Autodesk Inventor part; units mm, degrees
ref_plane "YZ Plane" through (0, 0, 0) normal (1, 0, 0) x (0, 1, 0)
ref_plane "XZ Plane" through (0, 0, 0) normal (0, 1, 0) x (-1, 0, 0)
ref_plane "XY Plane" through (0, 0, 0) normal (0, 0, 1) x (1, 0, 0)
sketch "Sketch1" plane through (0, 0, 0) normal (0, 1, 0) x (-1, 0, 0)
  line L0 (10.1226, -11.6524) -> (10.1226, 93.3476)
  line L1 (-18.8774, 93.3476) -> (-18.8774, -11.6524)
  line L2 (-18.8774, -11.6524) -> (-4.3774, -11.6524)
  line L3 (-4.3774, -11.6524) -> (-4.3774, 93.3476) construction
  line L4 (-18.8774, 40.8476) -> (-4.3774, 40.8476) construction
  line L5 (-18.8774, 93.3476) -> (10.1226, 93.3476)
  line L6 (-18.8774, 93.3476) -> (-9.8774, 93.3476)
  line L7 (-9.8774, 93.3476) -> (-9.8774, 99.3476)
  line L8 (-9.8774, 99.3476) -> (-18.8774, 99.3476)
  line L9 (-18.8774, 99.3476) -> (-18.8774, 93.3476)
  line L10 (10.1226, 93.3476) -> (1.1357, 93.3476)
  line L11 (1.1357, 93.3476) -> (1.1226, 99.3476)
  line L12 (1.1226, 99.3476) -> (10.1226, 99.3476)
  line L13 (10.1226, 99.3476) -> (10.1226, 93.3476)
  line L14 (-4.3774, 40.8476) -> (10.1226, 40.8476) construction
  line L15 (-4.3774, -11.6524) -> (10.1226, -11.6524)
  line L16 (-7.3774, 90.3476) -> (-16.3774, 90.3476)
  line L17 (-16.3774, 90.3476) -> (-16.3774, 84.3476)
  line L18 (-16.3774, 84.3476) -> (-7.3774, 84.3476)
  line L19 (-7.3774, 84.3476) -> (-7.3774, 90.3476)
  line L20 (-7.3774, 90.3476) -> (-16.3774, 84.3476) construction
  line L21 (-16.3774, 90.3476) -> (-7.3774, 84.3476) construction
  line L22 (-1.3774, 90.3476) -> (7.6226, 90.3476)
  line L23 (7.6226, 90.3476) -> (7.6226, 84.3476)
  line L24 (7.6226, 84.3476) -> (-1.3774, 84.3476)
  line L25 (-1.3774, 84.3476) -> (-1.3774, 90.3476)
  line L26 (-1.3774, 90.3476) -> (7.6226, 84.3476) construction
  line L27 (7.6226, 90.3476) -> (-1.3774, 84.3476) construction
  point P0 (-11.8774, 87.3476)
  point P1 (3.1226, 87.3476)
  dimension "d0" = 29
  dimension "d1" = 105
  dimension "d18" = 9
  dimension "d19" = 6
  dimension "d20" = 14.5
  dimension "d21" = 9
  dimension "d22" = 6
  dimension "d23" = 3
  dimension "d44" = 6
extrude "Extrusion1" add sketch "Sketch1" along normal blind 6
sketch "Sketch2" plane through (0, 6, 0) normal (0, 1, 0) x (1, 0, 0)
  line L0 (12.8733, -39.8476) -> (-6.1226, -39.8476) construction
  line L1 (-1.1357, -93.3476) -> (9.8774, -93.3476) construction
  line L2 (14.8774, -23.3476) -> (-6.1226, -23.3476) construction
  line L3 (14.8774, -21.8476) -> (-6.1226, -21.8476)
  line L4 (-6.1226, -24.8476) -> (14.8774, -24.8476)
  arc A0 (14.8774, -24.8476) -> (14.8774, -21.8476) centre (14.8774, -23.3476) ccw
  arc A1 (-6.1226, -21.8476) -> (-6.1226, -24.8476) centre (-6.1226, -23.3476) ccw
  line L5 (14.8774, -39.8476) -> (-6.1226, -39.8476) construction
  line L6 (14.8774, -38.3476) -> (-6.1226, -38.3476)
  line L7 (-6.1226, -41.3476) -> (14.8774, -41.3476)
  arc A2 (14.8774, -41.3476) -> (14.8774, -38.3476) centre (14.8774, -39.8476) ccw
  arc A3 (-6.1226, -38.3476) -> (-6.1226, -41.3476) centre (-6.1226, -39.8476) ccw
  line L8 (14.8774, -39.8476) -> (14.8774, -23.3476) construction
  line L9 (18.8774, -99.3476) -> (18.8774, 11.6524) construction
  line L10 (-10.1226, 11.6524) -> (-10.1226, -99.3476) construction
  line L11 (-6.1226, -39.8476) -> (-6.1226, -23.3476) construction
  point P0 (0, 0)
  point P1 (4.3747, -31.5976)
  point P2 (4.3774, -23.3476)
  point P3 (4.3774, -39.8476)
  point P4 (-6.1226, -31.5976)
  dimension "d46" = 3
  dimension "d47" = 3
  dimension "d48" = 16.5
  dimension "d49" = 70
  dimension "d50" = 4
  dimension "d51" = 4
extrude "Extrusion2" cut sketch "Sketch2" against normal through all
equation "\"d47\" = d46"
equation "\"d51\" = d50"
properties part number "thumper-bumper-sidewall-v3"
Can you work these out from the model? Positions are in its coordinate system, mm. A direction names the side the tool comes from. Give positions to 0.01 mm unless a question says otherwise; leave off trailing zeros. Loops run counter-clockwise (first coordinate to the right, second up) from the corner with the lowest first, then second, coordinate; pieces in that order, holes last. Notation, with made-up numbers: M -1,46 L 4,46 A34 ccw 4,85 Z; hole C -6,57.5 d11. An arc over 180 degrees is marked long. Use CSV: the item, a comma, the result in double quotes. Start each with the question number.
1. Imagine slicing it at A-A, the plane z = 88. Write out the boundary of the cut face in (x, y), plus the area to 3 significant figures.
2. Imagine slicing it at D-D, the plane x = -4.75. Write out the boundary of the cut face in (y, z).
3. Imagine slicing it at B-B, the plane y = 5. Write out the boundary of the cut face in (x, z), plus the area to 3 significant figures.
4. Imagine slicing it at C-C, the plane x = 3. Write out the boundary of the cut face in (y, z), plus the area to 3 significant figures.
5. If I drill on L1, parallel to Z at x = 8.25, y = 3.6; L2, parallel to Z at x = 4.25, y = 4.9; L3, parallel to Z at x = 13.25, y = 3.9, over which ranges is the centre line in solid material (lowest first)?
6. On a 3-axis mill with a long thin cutter (end or side, diameter ignored), from which of +Z, -Z, +X, -X, +Y, -Y can I reach the whole of each face in a straight line? I mean faces 1 (the face through (5, 3, 38.348)), 2 (the face through (4, 3, 93.348)), 3 (the face through (5, 3, -11.652)). Say none if no direction works.
7. For P1, Ø3, axis at x = 4.5, y = 3.5, coming from the +Z side, with a flat end and sliding along its axis, tell me the tip position at first contact or that it passes through.
8. If we mould it in two halves opening along X, with no side actions, what happens to faces 4 (the face through (14, 3, 99.348)), 5 (the face through (-3, 3, 84.348)), 6 (the face through (-10.123, 3, 43))? For each: released by +X, released by -X, zero draft, split by the parting line, or undercut.
Response values:
1,outline,"M -10.12,0 L -7.62,0 L -7.62,6 L -10.12,6 Z; M 1.38,0 L 7.38,0 L 7.38,6 L 1.38,6 Z; M 16.38,0 L 18.88,0 L 18.88,6 L 16.38,6 Z"
1,area,"66.0 mm^2"
2,outline,"M 0,-11.65 L 6,-11.65 L 6,21.85 L 0,21.85 Z; M 0,24.85 L 6,24.85 L 6,38.35 L 0,38.35 Z; M 0,41.35 L 6,41.35 L 6,84.35 L 0,84.35 Z; M 0,90.35 L 6,90.35 L 6,99.35 L 0,99.35 Z"
3,outline,"M -10.12,-11.65 L 18.88,-11.65 L 18.88,99.35 L 9.88,99.35 L 9.88,93.35 L -1.14,93.35 L -1.12,99.35 L -10.12,99.35 Z; hole M -7.62,84.35 L 1.38,84.35 L 1.38,90.35 L -7.62,90.35 Z; hole M -6.12,21.85 L 14.88,21.85 A1.5 ccw 14.88,24.85 L -6.12,24.85 A1.5 ccw Z; hole M -6.12,38.35 L 14.88,38.35 A1.5 ccw 14.88,41.35 L -6.12,41.35 A1.5 ccw Z; hole M 7.38,84.35 L 16.38,84.35 L 16.38,90.35 L 7.38,90.35 Z"
3,area,"2,900 mm^2"
4,outline,"M 0,-11.65 L 6,-11.65 L 6,21.85 L 0,21.85 Z; M 0,24.85 L 6,24.85 L 6,38.35 L 0,38.35 Z; M 0,41.35 L 6,41.35 L 6,93.35 L 0,93.35 Z"
4,area,"594 mm^2"
5,L1,"-11.65 to 21.85, 24.85 to 38.35, 41.35 to 84.35, 90.35 to 93.35"
5,L2,"-11.65 to 21.85, 24.85 to 38.35, 41.35 to 93.35"
5,L3,"-11.65 to 21.85, 24.85 to 38.35, 41.35 to 84.35, 90.35 to 99.35"
6,face 1,"+Y, -Y"
6,face 2,"+Z, +Y, -Y"
6,face 3,"-Z, +X, -X, +Y, -Y"
7,P1,"z = 93.35"
8,face 4,"zero draft"
8,face 5,"undercut"
8,face 6,"released by -X"
